The listing builds one solid part. Answer for the finished solid, in the listing's coordinates (mm). Give positions to 0.01 mm unless a question says otherwise; leave off trailing zeros. Write each loop counter-clockwise with the first axis right and the second up, starting at its lowest first coordinate (ties: lowest second). Pieces come first, ordered by that corner, then holes. Notation, with made-up numbers: (38.25, -29.5) -> (78.25, -29.5) arc R14 cw to (78.25, -7.5) -> close; hole circle Ø4 at (6, 36). An arc over 180 degrees is marked (long way). Put each result on its own line as item: value. Start each with the question number.
1) A cutting plane is placed at C-C (z = 5.5). Write down the section's boundary in (x, y).
2) Find the intervals of material crossed by line 1 along Y through (x, z) = (0, 16.5); line 2 along X through (y, z) = (-7.25, 24.25); line 3 along Y through (x, z) = (-14, 16), in increasing order. Write a range as from..to.
3) A cutting plane is placed at A-A (x = 0). Write down the section's boundary in (y, z), then the cut area to 3 significant figures.
4) A cutting plane is placed at B-B (y = 0). Write down the section's boundary in (x, z), then the cut area to 3 significant figures.
5) A cutting plane is placed at D-D (x = -13.5). Write down the section's boundary in (y, z).
6) Flat-ended cylindrical pins translate along their axes: pin 1 Ø2 at (y, z) = (6.5, 12.5) entering from -X (3 decimals); pin 2 Ø8 at (x, y) = (-0.5, 10) entering from -Z; pin 3 Ø10 at (y, z) = (-10.5, 5.5) entering from +X (3 decimals); pin 4 Ø5 at (y, z) = (9.5, 7) entering from +X. Find the tip coordinate at first contact, or state that the pin passes through.
from build123d import *

# Parameters (mm, degrees)
SCHIZZO2_R                   = 16
SCHIZZO2_R_2                 = 11
ESTRUSIONE_ESTRUSIONE1_DEPTH = 30
SCHIZZO3_W                   = 40.226432455
SCHIZZO3_H                   = 6.242620643
SCHIZZO3_W_2                 = 42.895225343
SCHIZZO3_H_2                 = 8.147240474
TAGLIO_ESTRUSIONE1_DEPTH     = 31


with BuildPart() as part:
    # Schizzo2 → Estrusione-Estrusione1 (new body)
    with BuildSketch(Plane.XY):
        Circle(SCHIZZO2_R)
        Circle(SCHIZZO2_R_2, mode=Mode.SUBTRACT)
    extrude(amount=ESTRUSIONE_ESTRUSIONE1_DEPTH)

    # Schizzo3 → Taglio-Estrusione1 (cut, through all)
    with BuildSketch(Plane.XY.offset(30)):
        with Locations((2.318761875, 17.121310322)):
            Rectangle(SCHIZZO3_W, SCHIZZO3_H)
        with Locations((2.584078566, -18.073620237)):
            Rectangle(SCHIZZO3_W_2, SCHIZZO3_H_2)
    extrude(amount=-TAGLIO_ESTRUSIONE1_DEPTH, mode=Mode.SUBTRACT)


solid = part.part
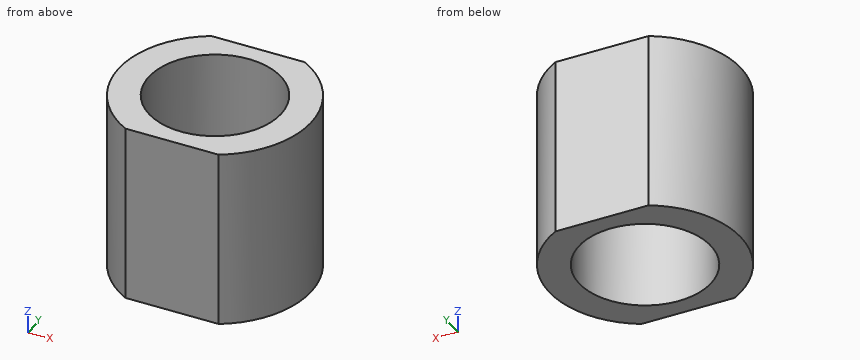
Reply:
1. outline: (-7.75, -14) -> (7.75, -14) arc R16 ccw to (7.75, 14) -> (-7.75, 14) arc R16 ccw to start; hole circle Ø22 at (0, 0)
2. line 1: y = -14..-11, 11..14
2. line 2: x = -14.26..-8.27, 8.27..14.26
2. line 3: y = -7.75..7.75
3. outline: (-14, 0) -> (-11, 0) -> (-11, 30) -> (-14, 30) -> close; (11, 0) -> (14, 0) -> (14, 30) -> (11, 30) -> close
3. area: 180 mm2
4. outline: (-16, 0) -> (-11, 0) -> (-11, 30) -> (-16, 30) -> close; (11, 0) -> (16, 0) -> (16, 30) -> (11, 30) -> close
4. area: 300 mm2
5. outline: (-8.59, 0) -> (8.59, 0) -> (8.59, 30) -> (-8.59, 30) -> close
6. pin 1: stops at x = -15.025
6. pin 2: stops at z = 0
6. pin 3: stops at x = 15.025
6. pin 4: stops at x = 14.39
